For this review, take the finished solid that the model builds, in its own axes (mm). A direction names the side the tool comes from. Give positions to 0.01 mm unless a question says otherwise; leave off trailing zeros. Order: outer loops, then holes, each group sorted by start corner. A loop starts at its lowest first (then second) coordinate and runs counter-clockwise, first axis right, second up. Notation, with made-up numbers: (-11, -40) - (30, -40) arc R16 cw to (30, -22) - close; hole circle Ø8 at (-31, -31). An arc over 180 degrees is marked (long way). Use a Markdown table: item, result. Add a question column.
1) We need section B-B on z = -47. Write out the cut boundary in (x, y), then the cut area to 3 significant figures.
2) Wall thickness on L1, parallel to Z at x = -65.5, y = 20; L2, parallel to X at y = 17, z = -57: over which ranges is each line inside the solid? List them lowest first.
3) Clearance check with flat-ended pins moving along their axes: P1, Ø8, axis at x = -66, y = 10.5, coming from the +Z side; P2, Ø1.5, axis at x = -162, z = -191.5, coming from the +Y side; P3, Ø8, axis at x = -103.5, z = -192, coming from the +Y side. State where each tip first meets the part, or that it passes through.
4) Mouldability with a two-part tool opening along Y and no side actions: class faces 1 (the face through (-26.26, 25.35, -169.96)), 2 (the face through (-47, 0, -183)), 3 (the face through (-52, 5, -195)) as released by +Y, released by -Y, zero draft, split by the parting line, or undercut.
5) We need section A-A on y = 42. Write out the cut boundary in (x, z).
6) Machinability: for faces 4 (the face through (-156, 25, -184.978)), 5 (the face through (5, 28, -63)), 6 (the face through (-156, 28, -189.978)), 7 (the face through (-23.236, 28.241, -173.944)), which of the approach directions +Z, -Z, +X, -X, +Y, -Y give a long, thin tool a straight path to every point of the face, cutting with its end or side? Answer none if there is none.
Autodesk Inventor part; units mm, degrees
ref_plane "YZ Plane" through (0, 0, 0) normal (1, 0, 0) x (0, 1, 0)
ref_plane "XZ Plane" through (0, 0, 0) normal (0, 1, 0) x (-1, 0, 0)
ref_plane "XY Plane" through (0, 0, 0) normal (0, 0, 1) x (1, 0, 0)
sketch "Эскиз1" plane through (0, 0, 0) normal (0, 0, 1) x (1, 0, 0)
  line L0 (0, 0) -> (0, 50)
  line L1 (0, 50) -> (2, 50)
  line L2 (5, 47) -> (5, 10)
  line L3 (10, 5) -> (47, 5)
  line L4 (50, 2) -> (50, 0)
  line L5 (50, 0) -> (0, 0)
  arc A0 (5, 47) -> (2, 50) centre (2, 47) ccw
  arc A1 (5, 10) -> (10, 5) centre (10, 10) ccw
  arc A2 (50, 2) -> (47, 5) centre (47, 2) ccw
  point P0 (5, 50)
  point P1 (5, 5)
  point P2 (50, 5)
  dimension "d6" = 50
  dimension "d7" = 5
  dimension "d8" = 45
  dimension "d9" = 45
  dimension "d10" = 3
  dimension "d11" = 5
  dimension "d12" = 3
sketch "Эскиз2" plane through (0, 0, 0) normal (0, 1, 0) x (-1, 0, 0)
  point P0 (0, 0)
sketch "Эскиз3" plane through (0, 0, 0) normal (0, 1, 0) x (-1, 0, 0)
  line L0 (0, 0) -> (0, -125.202)
  line L1 (19.7417, -165.0069) -> (32.6025, -174.7832)
  line L2 (62.8608, -184.9783) -> (246.0141, -184.9783)
  arc A0 (0, -125.202) -> (19.7417, -165.0069) centre (50, -125.202) ccw
  arc A1 (32.6025, -174.7832) -> (62.8608, -184.9783) centre (62.8608, -134.9783) ccw
  point P0 (0, -150)
  point P1 (46.0141, -184.9783)
  dimension "d13" = 150
  dimension "d14" = 200
  dimension "d15" = 50
sweep "Сдвиг1" add profiles "Эскиз1" path "Эскиз3"
properties part number "lab_4_3"
Checked values:
| question | item | result |
|---|---|---|
| 1 | outline | (0, 0) - (50, 0) - (50, 2) arc R3 ccw to (47, 5) - (10, 5) arc R5 cw to (5, 10) - (5, 47) arc R3 ccw to (2, 50) - (0, 50) - close |
| 1 | area | 477 mm² |
| 2 | L1 | -189.98 to -184.98 |
| 2 | L2 | 0 to 5 |
| 3 | P1 | z = -184.97 |
| 3 | P2 | y = 7.33 |
| 3 | P3 | y = 49.82 |
| 4 | face 1 | zero draft |
| 4 | face 2 | released by -Y |
| 4 | face 3 | released by +Y |
| 5 | outline | (-246.01, -189.98) - (-62.86, -189.98) arc R55 ccw to (-29.58, -178.76) - (-16.72, -168.99) arc R55 ccw to (5, -125.2) - (5, 0) - (0, 0) - (0, -125.2) arc R50 cw to (-19.74, -165.01) - (-32.6, -174.78) arc R50 cw to (-62.86, -184.98) - (-246.01, -184.98) - close |
| 6 | face 4 | +Z, -X, +Y, -Y |
| 6 | face 5 | +Z, -Z, +X, +Y |
| 6 | face 6 | -Z, +X, -X, +Y |
| 6 | face 7 | -Z, +X, +Y |
